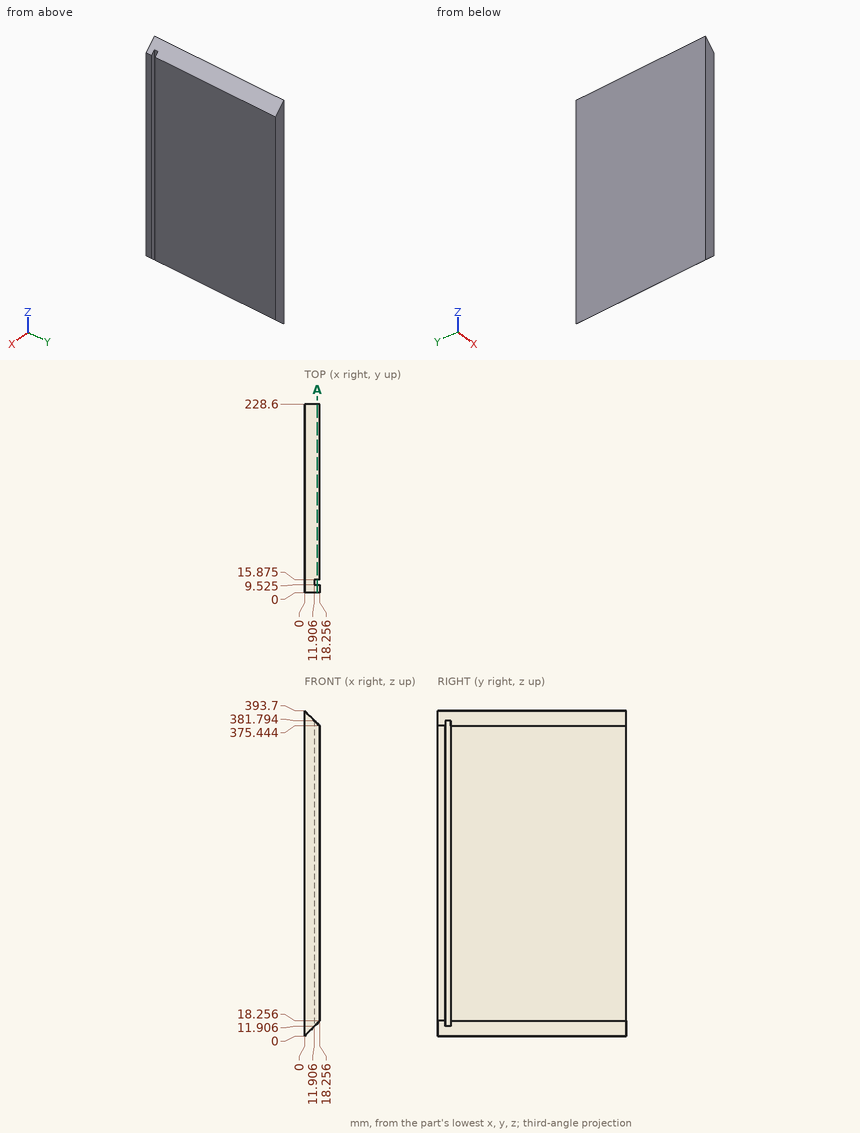
Answer from the drawing. Dimensions are ordinates in mm from the lowest x, y and z of the part. Give positions to 0.01 mm unless a question says otherwise; leave off trailing zeros. Order: outer loops, then holes, each group sorted by start corner. A loop starts at its lowest first (then second) coordinate and runs counter-clockwise, first axis right, second up. Notation, with made-up numbers: (70, -14) -> (124, -14) arc R11 ccw to (124, -8) -> close; hole circle Ø11 at (9, 83). An arc over 180 degrees is marked (long way). One line per item, written item: value. Start each with the question number.
(1) Flat-ended cylindrical pins translate along their axes: P1, Ø2, axis at y = 125.5, z = 318.5, coming from the -X side; P2, Ø4, axis at x = 13.5, y = 107.5, coming from the +Z side; P3, Ø8, axis at x = 7, y = 154, coming from the +Z side; P4, Ø5, axis at x = 5, y = 99.5, coming from the +Z side. Find the tip coordinate at first contact, or state that the pin passes through.
(2) Straight lines are drawn through the part: L1, parallel to Y at x = 16, z = 273.5 (1 decimal); L2, parallel to Z at x = 3, y = 31.5; L3, parallel to Z at x = 16.5, y = 26.5. For each, find the intervals that lie inside material, in ascending order.
(3) The part is cut by section A-A (x = 15.5). Determine the outline of the cut face in (y, z) (1 decimal), and give its area (3 significant figures).
Taken from the geometry:
1. P1: x = 0
1. P2: z = 382.2
1. P3: z = 390.7
1. P4: z = 391.2
2. L1: 0 to 9.5, 15.9 to 228.6
2. L2: 3 to 390.7
2. L3: 16.5 to 377.2
3. outline: (0, 15.5) -> (9.5, 15.5) -> (9.5, 378.2) -> (0, 378.2) -> close; (15.9, 15.5) -> (228.6, 15.5) -> (228.6, 378.2) -> (15.9, 378.2) -> close
3. area: 80,600 mm^2
